Work out the finished part from the listing and answer in its coordinate system (mm). Coordinates: 2 decimals unless noted, no trailing zeros. Order: outer loops, then holes, each group sorted by start corner. A loop starts at its lowest first (then second) coordinate and runs counter-clockwise, first axis right, second up. Notation, with made-up numbers: (71.5, -11.5) -> (83.5, -11.5) arc R5 cw to (83.5, -5.5) -> close; hole circle Ø3 at (59.25, 73.25). An arc over 180 degrees is marked (long way). Use one line per item in the form item = value.
from build123d import *

# Parameters (mm, degrees)
SKETCH1_W           = 6.858
SKETCH1_H           = 2.794
SKETCH1_R           = 1.27
BOSS_EXTRUDE1_DEPTH = 6.35


with BuildPart() as part:
    # Sketch1 → Boss-Extrude1 (new body)
    with BuildSketch(Plane(origin=(0, 0, 0), x_dir=(1, 0, 0), z_dir=(0, 1, 0))):
        Polygon((54.99261314, -31.75), (54.99261314, 31.75), (0, 63.5), (-54.99261314, 31.75), (-54.99261314, -31.75), (0, -63.5), align=None)
        with Locations((47.423090512, 18.923)):
            Rectangle(SKETCH1_W, SKETCH1_H, mode=Mode.SUBTRACT)
        with Locations((47.423090512, -18.923)):
            Rectangle(SKETCH1_W, SKETCH1_H, mode=Mode.SUBTRACT)
        Polygon((37.175006483, -29.337), (39.594681461, -27.94), (43.023681461, -33.879202219), (40.604006483, -35.276202219), align=None, mode=Mode.SUBTRACT)
        Polygon((4.399409051, -48.26), (6.819084029, -46.863), (10.248084029, -52.802202219), (7.828409051, -54.199202219), align=None, mode=Mode.SUBTRACT)
        Polygon((-6.819084029, -46.863), (-4.399409051, -48.26), (-7.828409051, -54.199202219), (-10.248084029, -52.802202219), align=None, mode=Mode.SUBTRACT)
        Polygon((-39.594681461, -27.94), (-37.175006483, -29.337), (-40.604006483, -35.276202219), (-43.023681461, -33.879202219), align=None, mode=Mode.SUBTRACT)
        with Locations((-47.423090512, -18.923)):
            Rectangle(SKETCH1_W, SKETCH1_H, mode=Mode.SUBTRACT)
        with Locations((-47.423090512, 18.923)):
            Rectangle(SKETCH1_W, SKETCH1_H, mode=Mode.SUBTRACT)
        Polygon((-37.175006483, 29.337), (-39.594681461, 27.94), (-43.023681461, 33.879202219), (-40.604006483, 35.276202219), align=None, mode=Mode.SUBTRACT)
        Polygon((-4.399409051, 48.26), (-6.819084029, 46.863), (-10.248084029, 52.802202219), (-7.828409051, 54.199202219), align=None, mode=Mode.SUBTRACT)
        Polygon((6.819084029, 46.863), (4.399409051, 48.26), (7.828409051, 54.199202219), (10.248084029, 52.802202219), align=None, mode=Mode.SUBTRACT)
        Polygon((39.594681461, 27.94), (37.175006483, 29.337), (40.604006483, 35.276202219), (43.023681461, 33.879202219), align=None, mode=Mode.SUBTRACT)
        with Locations(Location((0, 0, 0), (0, 0, 270))):
            Circle(SKETCH1_R, mode=Mode.SUBTRACT)
    extrude(amount=BOSS_EXTRUDE1_DEPTH)


solid = part.part
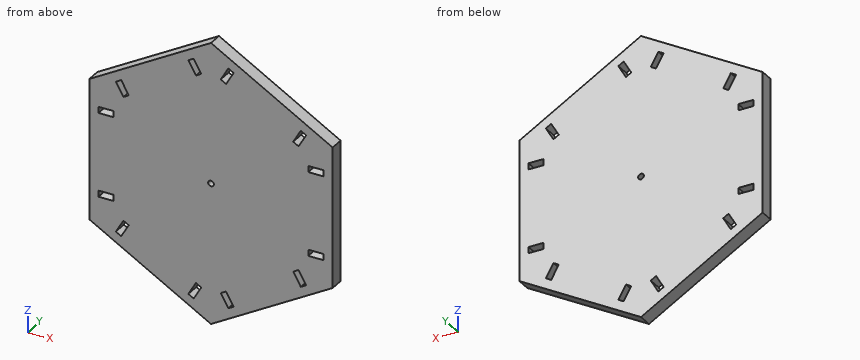
(1) Section C-C on x = -17 is taken. Write down the section's boundary in (y, z).
Data:
outline = (0, -53.69) -> (6.35, -53.69) -> (6.35, 53.69) -> (0, 53.69) -> close
(2) Section B-B on y = 3 is taken. Count the separate pieces of the cut face and the enclosed holes in it, plus the area to 3 significant figures.
Data:
separate_pieces = 1
enclosed_holes = 13
area = 10,200 mm²
(3) Straight lines are drawn through the part: line 1 along X through (y, z) = (3.5, 0); line 2 along X through (y, z) = (2, -29); line 3 along X through (y, z) = (3, 47). For each, find the intervals that lie inside material, in ascending order.
Data:
line_1 = -54.99 to -1.27, 1.27 to 54.99
line_2 = -54.99 to -40.21, -37.76 to 37.76, 40.21 to 54.99
line_3 = -28.58 to -6.9, -6.58 to 6.58, 6.9 to 28.58
(4) Section A-A on x = -47 is taken. Write down the section's boundary in (y, z), plus the area to 3 significant figures.
Data:
outline = (0, -36.36) -> (6.35, -36.36) -> (6.35, -20.32) -> (0, -20.32) -> close; (0, -17.53) -> (6.35, -17.53) -> (6.35, 17.53) -> (0, 17.53) -> close; (0, 20.32) -> (6.35, 20.32) -> (6.35, 36.36) -> (0, 36.36) -> close
area = 426 mm²
(5) Each of these flat-tipped pins is pushed along its axis until it touches: P1, Ø3, axis at x = 46, y = 2.5, coming from the +Z side; P2, Ø2, axis at x = 2.5, y = 4, coming from the +Z side; P3, Ø3, axis at x = 47, y = 2.5, coming from the +Z side; P4, Ø1.5, axis at x = 0, z = 0, coming from the -Y side. Where does it stop, or does it pass through?
Data:
P1 = 37.81
P2 = 62.63
P3 = 37.23
P4 = through
